from build123d import *

# Parameters (mm, degrees)
SKETCH_1_W                   = 14
SKETCH_1_H                   = 35
EXTRUDE_1_DEPTH              = 7
HOLE_WIZARD_M6_1_D           = 7
HOLE_WIZARD_M6_1_CSINK_D     = 12.8
HOLE_WIZARD_M6_1_CSINK_ANGLE = 90
SKETCH_6_W                   = 7
SKETCH_6_H                   = 35
EXTRUDE_2_DEPTH              = 38
SKETCH_7_R                   = 5.5
EXTRUDE_3_DEPTH              = 7


with BuildPart() as part:
    # 草图1 → 凸台-拉伸1 (new body)
    with BuildSketch(Plane(origin=(0, 0, 0), x_dir=(1, 0, 0), z_dir=(0, 1, 0))):
        Rectangle(SKETCH_1_W, SKETCH_1_H)
    extrude(amount=EXTRUDE_1_DEPTH)

    # M6 内六角花形半沉头螺钉的锥形沉头孔1 (through all)
    with Locations(Plane(origin=(0, 7, 0), x_dir=(1, 0, 0), z_dir=(0, 1, 0))):
        with Locations((0, -9), (0, 9)):
            CounterSinkHole(HOLE_WIZARD_M6_1_D / 2, HOLE_WIZARD_M6_1_CSINK_D / 2, counter_sink_angle=HOLE_WIZARD_M6_1_CSINK_ANGLE)

    # 草图6 → 凸台-拉伸2 (add)
    with BuildSketch(Plane(origin=(0, 0, 0), x_dir=(1, 0, 0), z_dir=(0, 1, 0))):
        with Locations((10.5, 0)):
            Rectangle(SKETCH_6_W, SKETCH_6_H)
    extrude(amount=EXTRUDE_2_DEPTH)

    # 草图7 → 凸台-拉伸3 (add)
    with BuildSketch(Plane.XY.offset(17.5)):
        with BuildLine():
            Line((14, 38), (26, 38))
            ThreePointArc((26, 38), (37, 27), (26, 16))
            Line((26, 16), (14, 16))
            Line((14, 16), (14, 38))
        make_face()
        with Locations((26, 27)):
            Circle(SKETCH_7_R, mode=Mode.SUBTRACT)
    extrude_3 = extrude(amount=-EXTRUDE_3_DEPTH)

    # 镜向1: 凸台-拉伸3 across plane
    add(extrude_3.mirror(Plane.XY))


solid = part.part
Can you work these out from the model? Positions are in its coordinate system, mm. A direction names the side the tool comes from. Round coordinates to 2 decimals unless told otherwise and drop trailing zeros. Write each loop counter-clockwise with the first axis right and the second up, starting at its lowest first coordinate (ties: lowest second). Pieces come first, ordered by that corner, then holes. Notation, with made-up numbers: (-3, 60) -> (14, 60) arc R26 cw to (14, 84) -> close; hole circle Ø2 at (2.25, 89). An arc over 180 degrees is marked (long way). One line per question, with ' | ' between items. Start each with the question number.
1) Suppose I cut it at B-B on y = 27. Write out the boundary of the cut face in (x, z), then the cut area to 3 significant figures.
2) Suppose I cut it at C-C on z = 9. Write out the boundary of the cut face in (x, y), then the cut area to 3 significant figures.
3) If we mould it in two halves opening along Z, with no side actions, what happens to faces 1 (the flat face through (15, 19, -17.5)), 2 (the flat face through (15, 19, 17.5)), 3 (the flat face through (14, 15, 0)), 4 (the flat face through (3, 0, 0))? For each: released by +Z, released by -Z, zero draft, split by the parting line, or undercut.
4) On a 3-axis mill with a long thin cutter (end or side, diameter ignored), from which of +Z, -Z, +X, -X, +Y, -Y can I reach the whole of each face in a straight line? I mean faces 5 (the flat face through (0, 7, 0)), 6 (the flat face through (20.5, 24.7, -10.5)), 7 (the flat face through (20, 16, -14)). Say none if no direction works.
5) I'm going to push flat-ended pins straight in: P1, Ø8, axis at y = 21, z = 9.5, coming from the -X side; P2, Ø5.5, axis at x = 22.5, z = 14, coming from the -Y side; P3, Ø10, axis at x = 26, y = 27, coming from the +Z side. Where does each tip first touch, or does it pass through?
6) Suppose I cut it at D-D on x = 0. Write out the boundary of the cut face in (y, z), then the cut area to 3 significant figures.
7) I need wall thicknesses on line 1 (Z direction, x = 0, y = 2.15); line 2 (Y direction, x = 26, z = -12.25); line 3 (Z direction, x = 28, y = 33.5). Which ranges of each line are inside material? Lowest first, please. Write a range as [from, to].
8) Suppose I cut it at A-A on x = 16. Write out the boundary of the cut face in (y, z), then the cut area to 3 significant figures.
Return value:
1) outline: (7, -17.5) -> (20.5, -17.5) -> (20.5, -10.5) -> (14, -10.5) -> (14, 10.5) -> (20.5, 10.5) -> (20.5, 17.5) -> (7, 17.5) -> close; (31.5, -17.5) -> (37, -17.5) -> (37, -10.5) -> (31.5, -10.5) -> close; (31.5, 10.5) -> (37, 10.5) -> (37, 17.5) -> (31.5, 17.5) -> close | area: 413 mm2
2) outline: (-7, 0) -> (-3.5, 0) -> (-3.5, 4.1) -> (-6.4, 7) -> (-7, 7) -> close; (3.5, 0) -> (14, 0) -> (14, 38) -> (7, 38) -> (7, 7) -> (6.4, 7) -> (3.5, 4.1) -> close | area: 307 mm2
3) face 1: released by -Z | face 2: released by +Z | face 3: undercut | face 4: zero draft
4) face 5: +Z, -Z, -X, +Y | face 6: +X, +Y, -Y | face 7: +Z, -Z, +X, -Y
5) P1: stops at x = 7 | P2: stops at y = 16 | P3: passes through
6) outline: (0, -17.5) -> (7, -17.5) -> (7, -15.4) -> (4.1, -12.5) -> (0, -12.5) -> close; (0, -5.5) -> (4.1, -5.5) -> (7, -2.6) -> (7, 2.6) -> (4.1, 5.5) -> (0, 5.5) -> close; (0, 12.5) -> (4.1, 12.5) -> (7, 15.4) -> (7, 17.5) -> (0, 17.5) -> close | area: 130 mm2
7) line 1: z = [-17.5, -12.5], [-5.5, 5.5], [12.5, 17.5] | line 2: y = [16, 21.5], [32.5, 38] | line 3: z = [-17.5, -10.5], [10.5, 17.5]
8) outline: (16, -17.5) -> (38, -17.5) -> (38, -10.5) -> (16, -10.5) -> close; (16, 10.5) -> (38, 10.5) -> (38, 17.5) -> (16, 17.5) -> close | area: 308 mm2
